Model file for the job. Use its own axes, mm. A direction names the side the tool comes from. Give positions to 0.01 mm unless a question says otherwise; leave off trailing zeros. Write each loop counter-clockwise with the first axis right and the second up, starting at its lowest first coordinate (ties: lowest second). Pieces come first, ordered by that corner, then holes.
```python
from build123d import *

# Parameters (mm, degrees)
SKETCH1_W           = 6
SKETCH1_H           = 17
BOSS_EXTRUDE1_DEPTH = 1.2
SKETCH2_W           = 2
SKETCH2_H           = 17
BOSS_EXTRUDE2_DEPTH = 68
CUT_EXTRUDE1_REACH  = 72.337
SKETCH3_W           = 0.8
SKETCH3_H           = 0.8
SKETCH3_W_2         = 10
SKETCH3_H_2         = 0.5
CUT_EXTRUDE3_REACH  = 72.337
SKETCH4_W           = 17
SKETCH4_H           = 17.2
SKETCH4_W_2         = 6.6
SKETCH4_H_2         = 16.4
SKETCH4_H_3         = 16.6
CUT_EXTRUDE4_REACH  = 61.352
SKETCH5_W           = 0.8
SKETCH5_H           = 17


with BuildPart() as part:
    # Sketch1 → Boss-Extrude1 (new body)
    with BuildSketch(Plane(origin=(0, 0, 0), x_dir=(1, 0, 0), z_dir=(0, 1, 0))):
        with Locations((-23, 3.444444444)):
            Rectangle(SKETCH1_W, SKETCH1_H)
    extrude(amount=BOSS_EXTRUDE1_DEPTH)

    # Sketch2 → Boss-Extrude2 (add)
    with BuildSketch(Plane(origin=(0, 1.2, 0), x_dir=(1, 0, 0), z_dir=(0, 1, 0))):
        with Locations((-25, 3.444444444)):
            Rectangle(SKETCH2_W, SKETCH2_H)
    extrude(amount=BOSS_EXTRUDE2_DEPTH)

    # Sketch3 → Cut-Extrude1 (cut, up to next)
    with BuildSketch(Plane(origin=(-24, 0, 0), x_dir=(0, 0, -1), z_dir=(1, 0, 0)), mode=Mode.PRIVATE) as cut_extrude1_sk1:
        with Locations((3.444444444, 23.8)):
            Rectangle(SKETCH3_W, SKETCH3_H)
    cut_extrude1_tool1 = extrude(cut_extrude1_sk1.sketch, amount=-CUT_EXTRUDE1_REACH, mode=Mode.PRIVATE) & part.part
    # Sketch3 → Cut-Extrude1 (cut, up to next)
    with BuildSketch(Plane(origin=(-24, 0, 0), x_dir=(0, 0, -1), z_dir=(1, 0, 0)), mode=Mode.PRIVATE) as cut_extrude1_sk2:
        with Locations((3.444444444, 46.6)):
            Rectangle(SKETCH3_W, SKETCH3_H)
    cut_extrude1_tool2 = extrude(cut_extrude1_sk2.sketch, amount=-CUT_EXTRUDE1_REACH, mode=Mode.PRIVATE) & part.part
    # Sketch3 → Cut-Extrude1 (cut, up to next)
    with BuildSketch(Plane(origin=(-24, 0, 0), x_dir=(0, 0, -1), z_dir=(1, 0, 0)), mode=Mode.PRIVATE) as cut_extrude1_sk3:
        with Locations((3.444444444, 22.85)):
            Rectangle(SKETCH3_W_2, SKETCH3_H_2)
    cut_extrude1_tool3 = extrude(cut_extrude1_sk3.sketch, amount=-CUT_EXTRUDE1_REACH, mode=Mode.PRIVATE) & part.part
    # Sketch3 → Cut-Extrude1 (cut, up to next)
    with BuildSketch(Plane(origin=(-24, 0, 0), x_dir=(0, 0, -1), z_dir=(1, 0, 0)), mode=Mode.PRIVATE) as cut_extrude1_sk4:
        with Locations((3.444444444, 45.65)):
            Rectangle(SKETCH3_W_2, SKETCH3_H_2)
    cut_extrude1_tool4 = extrude(cut_extrude1_sk4.sketch, amount=-CUT_EXTRUDE1_REACH, mode=Mode.PRIVATE) & part.part
    add(cut_extrude1_tool1.solids().sort_by_distance((-24, 23.8, -3.444444))[0], mode=Mode.SUBTRACT)
    add(cut_extrude1_tool2.solids().sort_by_distance((-24, 46.6, -3.444444))[0], mode=Mode.SUBTRACT)
    add(cut_extrude1_tool3.solids().sort_by_distance((-24, 22.85, -3.444444))[0], mode=Mode.SUBTRACT)
    add(cut_extrude1_tool4.solids().sort_by_distance((-24, 45.65, -3.444444))[0], mode=Mode.SUBTRACT)

    # Sketch4 → Cut-Extrude3 (cut, up to next)
    with BuildSketch(Plane(origin=(-24, 0, 0), x_dir=(0, 0, -1), z_dir=(1, 0, 0)), mode=Mode.PRIVATE) as cut_extrude3_sk1:
        with Locations((3.444444444, 60.6)):
            Rectangle(SKETCH4_W, SKETCH4_H)
    cut_extrude3_tool1 = extrude(cut_extrude3_sk1.sketch, amount=-CUT_EXTRUDE3_REACH, mode=Mode.PRIVATE) & part.part
    # Sketch4 → Cut-Extrude3 (cut, up to next)
    with BuildSketch(Plane(origin=(-24, 0, 0), x_dir=(0, 0, -1), z_dir=(1, 0, 0)), mode=Mode.PRIVATE) as cut_extrude3_sk2:
        with Locations((3.444444444, 34.8)):
            Rectangle(SKETCH4_W_2, SKETCH4_H_2)
    cut_extrude3_tool2 = extrude(cut_extrude3_sk2.sketch, amount=-CUT_EXTRUDE3_REACH, mode=Mode.PRIVATE) & part.part
    # Sketch4 → Cut-Extrude3 (cut, up to next)
    with BuildSketch(Plane(origin=(-24, 0, 0), x_dir=(0, 0, -1), z_dir=(1, 0, 0)), mode=Mode.PRIVATE) as cut_extrude3_sk3:
        with Locations((3.444444444, 11.9)):
            Rectangle(SKETCH4_W_2, SKETCH4_H_3)
    cut_extrude3_tool3 = extrude(cut_extrude3_sk3.sketch, amount=-CUT_EXTRUDE3_REACH, mode=Mode.PRIVATE) & part.part
    add(cut_extrude3_tool1.solids().sort_by_distance((-24, 60.6, -3.444444))[0], mode=Mode.SUBTRACT)
    add(cut_extrude3_tool2.solids().sort_by_distance((-24, 34.8, -3.444444))[0], mode=Mode.SUBTRACT)
    add(cut_extrude3_tool3.solids().sort_by_distance((-24, 11.9, -3.444444))[0], mode=Mode.SUBTRACT)

    # Cut-Extrude4: up to this face of the body (flat: up to its plane)
    cut_extrude4_end = Plane(part.part.faces().sort_by_distance((-22, 1.2, -3.444444444))[0])
    # Sketch5 → Cut-Extrude4 (cut, up to the picked face)
    with BuildSketch(Plane(origin=(0, 52, 0), x_dir=(1, 0, 0), z_dir=(0, 1, 0)), mode=Mode.PRIVATE) as cut_extrude4_sk1:
        with Locations((-24.4, 3.444444444)):
            Rectangle(SKETCH5_W, SKETCH5_H)
    cut_extrude4_tool1 = split(extrude(cut_extrude4_sk1.sketch, amount=-CUT_EXTRUDE4_REACH, mode=Mode.PRIVATE), bisect_by=cut_extrude4_end, keep=Keep.BOTH, mode=Mode.PRIVATE)
    add(cut_extrude4_tool1.solids().sort_by(Axis((-24.4, 52, -3.444444), (0, -1, 0)))[0], mode=Mode.SUBTRACT)


solid = part.part
```
1. Slice it at A-A, the plane y = 31.5. Write the cut outline in (x, z), and give its area (3 significant figures).
Calculated:
outline: (-26, -11.94) - (-24.8, -11.94) - (-24.8, -6.74) - (-26, -6.74) - close; (-26, -0.14) - (-24.8, -0.14) - (-24.8, 5.06) - (-26, 5.06) - close
area: 12.5 mm2
2. Slice it at B-B, the plane z = -4.75. Write the cut outline in (x, y).
Calculated:
outline: (-26, 0) - (-20, 0) - (-20, 1.2) - (-24.8, 1.2) - (-24.8, 3.6) - (-26, 3.6) - close; (-26, 20.2) - (-24.8, 20.2) - (-24.8, 22.6) - (-26, 22.6) - close; (-26, 23.1) - (-24.8, 23.1) - (-24.8, 26.6) - (-26, 26.6) - close; (-26, 43) - (-24.8, 43) - (-24.8, 45.4) - (-26, 45.4) - close; (-26, 45.9) - (-24.8, 45.9) - (-24.8, 52) - (-26, 52) - close
3. Which spindle directions (+Z, -Z, +X, -X, +Y, -Y) get a long thin tool onto all of the face, cutting with end or side? Do faces 1 (the flat face through (-24.8, 27, -7)), 2 (the flat face through (-25, 45.4, -3)), 3 (the flat face through (-25, 52, -3)). Say none if no direction does.
Calculated:
face 1: +Z, -Z, +X, +Y
face 2: +X, -X
face 3: +Z, -Z, +X, -X, +Y
4. Pull direction Z, two halves, no side cores. Call faces 4 (the flat face through (-25, 43, -3)), 5 (the flat face through (-25, 22, -11.944)), 6 (the flat face through (-25, 3.6, -3)), 7 (the flat face through (-22, 1.2, -4)): +Z half, -Z half, draft (parallel to the pull), parting line (faces both ways), or undercut.
Calculated:
face 4: undercut
face 5: -Z half
face 6: undercut
face 7: draft
5. Slice it at D-D, the plane x = -21.25. Write the cut outline in (y, z).
Calculated:
outline: (0, -11.94) - (1.2, -11.94) - (1.2, 5.06) - (0, 5.06) - close
6. Pin check, flat tip, straight feed: P1, Ø6, axis at y = 11, z = 2.5, coming from the +X side. Stop position of the tip, or through.
Calculated:
P1: stops at x = -24.8
7. Probe probe 1 along Y at (x, z) = (-25.05, -1); probe 2 along Z at (x, y) = (-25.5, 30); probe 3 along X at (y, z) = (37, -7). List the from-to ranges inside material, lowest first.
Calculated:
probe 1: y = 0 to 3.6, 20.2 to 22.6, 23.1 to 26.6, 43 to 45.4, 45.9 to 52
probe 2: z = -11.94 to -6.74, -0.14 to 5.06
probe 3: x = -26 to -24.8
8. Slice it at C-C, the plane z = 3.5. Write the cut outline in (x, y), and give its area (3 significant figures).
Calculated:
outline: (-26, 0) - (-20, 0) - (-20, 1.2) - (-24.8, 1.2) - (-24.8, 52) - (-26, 52) - close
area: 68.2 mm2
